from build123d import *

# Parameters (mm, degrees)
ESBO_O1_W                = 50
ESBO_O1_H                = 20
RESSALTO_EXTRUS_O1_DEPTH = 2.5
ESBO_O2_R                = 2.6
CORTE_EXTRUS_O1_DEPTH    = 6
FILETE1_R                = 5


with BuildPart() as part:
    # Esboço1 → Ressalto-extrusão1 (new, symmetric)
    with BuildSketch(Plane(origin=(0, 0, 0), x_dir=(1, 0, 0), z_dir=(0, 1, 0))):
        Rectangle(ESBO_O1_W, ESBO_O1_H)
    extrude(amount=RESSALTO_EXTRUS_O1_DEPTH, both=True)

    # Esboço2 → Corte-extrusão1 (cut)
    with BuildSketch(Plane(origin=(0, 2.5, 0), x_dir=(1, 0, 0), z_dir=(0, 1, 0))):
        with Locations(Location((-15, 0, 0), (0, 0, 270))):
            Circle(ESBO_O2_R)
        with Locations(Location((15, 0, 0), (0, 0, 270))):
            Circle(ESBO_O2_R)
    extrude(amount=-CORTE_EXTRUS_O1_DEPTH, mode=Mode.SUBTRACT)

    # Filete1
    filete1_edges = [part.edges().sort_by_distance(p)[0] for p in [
        (25, 0, 10),
        (-25, 0, 10),
        (-25, 0, -10),
        (25, 0, -10),
    ]]
    fillet(filete1_edges, radius=FILETE1_R)


solid = part.part
The listing builds one solid part. Answer for the finished solid, in the listing's coordinates (mm). Give positions to 0.01 mm unless a question says otherwise; leave off trailing zeros. Order: outer loops, then holes, each group sorted by start corner. A loop starts at its lowest first (then second) coordinate and runs counter-clockwise, first axis right, second up. Notation, with made-up numbers: (20, 77.25) - (48, 77.25) arc R27 ccw to (48, 101.25) - close; hole circle Ø3 at (-20, 41). An arc over 180 degrees is marked (long way). One line per item, written item: value. Start each with the question number.
1) A cutting plane is placed at B-B on x = 15. Give the vertices of the cut face in (y, z).
2) A cutting plane is placed at D-D on x = -17. Give the vertices of the cut face in (y, z), then the cut area to 3 significant figures.
3) A cutting plane is placed at A-A on z = 0. Give the vertices of the cut face in (x, y).
4) The mould has two halves that part along Z. Classify faces 1 (the face through (-17.54, 0.04, -0.56)), 2 (the face through (0, 0, -10)), 3 (the face through (0, 2.5, 0)): released by +Z, released by -Z, zero draft, split by the parting line, or undercut.
5) Find the intervals of material crossed by L1, parallel to X at y = 1.3, z = 0; L2, parallel to X at y = 0.4, z = -1; L3, parallel to Z at x = 16, y = 0.4, in increasing order.
6) A cutting plane is placed at C-C on y = 1.05. Give the vertices of the cut face in (x, z), then the cut area to 3 significant figures.
Answer sheet:
1. outline: (-2.5, -10) - (2.5, -10) - (2.5, -2.6) - (-2.5, -2.6) - close; (-2.5, 2.6) - (2.5, 2.6) - (2.5, 10) - (-2.5, 10) - close
2. outline: (-2.5, -10) - (2.5, -10) - (2.5, -1.66) - (-2.5, -1.66) - close; (-2.5, 1.66) - (2.5, 1.66) - (2.5, 10) - (-2.5, 10) - close
2. area: 83.4 mm2
3. outline: (-25, -2.5) - (-17.6, -2.5) - (-17.6, 2.5) - (-25, 2.5) - close; (-12.4, -2.5) - (12.4, -2.5) - (12.4, 2.5) - (-12.4, 2.5) - close; (17.6, -2.5) - (25, -2.5) - (25, 2.5) - (17.6, 2.5) - close
4. face 1: undercut
4. face 2: released by -Z
4. face 3: zero draft
5. L1: x = -25 to -17.6, -12.4 to 12.4, 17.6 to 25
5. L2: x = -25 to -17.4, -12.6 to 12.6, 17.4 to 25
5. L3: z = -10 to -2.4, 2.4 to 10
6. outline: (-25, -5) arc R5 ccw to (-20, -10) - (20, -10) arc R5 ccw to (25, -5) - (25, 5) arc R5 ccw to (20, 10) - (-20, 10) arc R5 ccw to (-25, 5) - close; hole circle Ø5.2 at (-15, 0); hole circle Ø5.2 at (15, 0)
6. area: 936 mm2
